```python
from build123d import *

# Parameters (mm, degrees)
SKETCH_1_R        = 80
SKETCH_1_R_2      = 43
EXTRUDE_1_DEPTH   = 70
SKETCH_1_R_3      = 50
SKETCH_1_R_4      = 22.5
EXTRUDE_1_2_DEPTH = 70
EXTRUDE_START     = -52.5
EXTRUDE_2_DEPTH   = 35


with BuildPart() as part:
    # Sketch 1 → Extrude 1 (new body)
    with BuildSketch(Plane(origin=(0, 0, 0), x_dir=(1, 0, 0), z_dir=(0, 1, 0))):
        with Locations(Location((-122.899042893, 0, 0), (0, 0, 270))):
            Circle(SKETCH_1_R)
        with Locations(Location((-122.899042893, 0, 0), (0, 0, 270))):
            Circle(SKETCH_1_R_2, mode=Mode.SUBTRACT)
    extrude(amount=EXTRUDE_1_DEPTH)



with BuildPart() as body_2:
    # Sketch 1 → Extrude 1 2 (new body)
    with BuildSketch(Plane(origin=(0, 0, 0), x_dir=(1, 0, 0), z_dir=(0, 1, 0))):
        with Locations(Location((107.100957107, 0, 0), (0, 0, 270))):
            Circle(SKETCH_1_R_3)
        with Locations(Location((107.100957107, 0, 0), (0, 0, 270))):
            Circle(SKETCH_1_R_4, mode=Mode.SUBTRACT)
    extrude(amount=EXTRUDE_1_2_DEPTH)


with BuildPart() as part_1:
    add(part.part)

    add(body_2.part)  # Extrude 2 merges body 2
    # Sketch 2 → Extrude 2 (add)
    with BuildSketch(Plane(origin=(0, 70, 0), x_dir=(1, 0, 0), z_dir=(0, 1, 0)).offset(EXTRUDE_START)):
        with BuildLine():
            Line((-112.464260284, 79.316551311), (113.622696237, 49.57284457))
            ThreePointArc((113.622696237, 49.57284457), (61.083229888, 19.554252264), (75.941536817, -39.10358714))
            ThreePointArc((75.941536817, -39.10358714), (4.230318414, -17.752822315), (-62.222714391, -52.138116186))
            ThreePointArc((-62.222714391, -52.138116186), (-48.171003091, 28.560813493), (-112.464260284, 79.316551311))
        make_face()
    extrude(amount=EXTRUDE_2_DEPTH)


solid = part_1.part
```
The listing builds one solid part. Answer for the finished solid, in the listing's coordinates (mm). A direction names the side the tool comes from. Coordinates: 2 decimals unless noted, no trailing zeros. Loops run counter-clockwise (first coordinate to the right, second up) from the corner with the lowest first, then second, coordinate; pieces in that order, holes last. Notation, with made-up numbers: (61, 16.25) -> (89, 16.25) arc R22 ccw to (89, 30.25) -> close; hole circle Ø6 at (5, 66.25). An arc over 180 degrees is marked (long way). Use one line per item in the form item = value. Start each with the question number.
Item 1: Consider L1, parallel to X at y = 47, z = 0; L2, parallel to X at y = 13, z = 5; L3, parallel to Z at x = 132.5, y = 61. Determine where each line is inside the solid, lowest interval first. Write a range as [from, to].
Item 2: The part is cut by section C-C on y = 60. Determine the outline of the cut face in (x, z), then the cut area to 3 significant figures.
Item 3: Flat-ended cylindrical pins translate along their axes: pin 1 Ø8 at (x, y) = (-107.5, 12.5) entering from +Z; pin 2 Ø1 at (y, z) = (16, -45.5) entering from -X; pin 3 Ø6 at (y, z) = (23.5, -52) entering from -X; pin 4 Ø5 at (x, z) = (104, -55) entering from -Y. Find the tip coordinate at first contact, or state that the pin passes through.
Item 4: The mould has two halves that part along X. Classify faces 1 (the face through (-1.003, 34.755, -64.653)), 2 (the face through (-157, 0, 34)), 3 (the face through (1, 17.5, -24)): released by +X, released by -X, zero draft, split by the parting line, or undercut.
Item 5: The part is cut by section D-D on z = -60.5. Determine the outline of the cut face in (x, y), then the cut area to 3 significant figures.
Item 6: The part is cut by section B-B on x = 124. Determine the outline of the cut face in (y, z), then the cut area to 3 significant figures.
Item 7: A tool of negligible diameter and unlimited length cuts with its end or side. For faces 4 (the face through (149.26, 34.51, 26.88)), 5 (the face through (5.3, 34.755, 17.658)), from which of +Z, -Z, +X, -X, +Y, -Y can it reach the whole face along a straight path? Write none if from no direction.
Item 8: The part is cut by section A-A on z = 0. Determine the outline of the cut face in (x, y).
Answer key:
q1.L1 = [-202.9, -165.9], [-79.9, 84.6], [129.6, 157.1]
q1.L2 = [-202.74, -165.61], [-80.19, -43.06], [57.35, 85.16], [129.04, 156.85]
q1.L3 = [-43.07, 43.07]
q2.outline = circle Ø160 at (-122.9, 0); circle Ø100 at (107.1, 0); hole circle Ø86 at (-122.9, 0); hole circle Ø45 at (107.1, 0)
q2.area = 20,600 mm2
q3.pin_1 = 79.18
q3.pin_2 = -189.04
q3.pin_3 = -186.14
q3.pin_4 = through
q4.face_1 = released by +X
q4.face_2 = zero draft
q4.face_3 = undercut
q5.outline = (-175.24, 0) -> (-70.56, 0) -> (-70.56, 17.5) -> (30.56, 17.5) -> (30.56, 52.5) -> (-70.56, 52.5) -> (-70.56, 70) -> (-175.24, 70) -> close
q5.area = 10,900 mm2
q6.outline = (0, -47.06) -> (70, -47.06) -> (70, -14.86) -> (0, -14.86) -> close; (0, 14.86) -> (70, 14.86) -> (70, 47.06) -> (0, 47.06) -> close
q6.area = 4,510 mm2
q7.face_4 = none
q7.face_5 = +Z, +Y, -Y
q8.outline = (-202.9, 0) -> (-165.9, 0) -> (-165.9, 70) -> (-202.9, 70) -> close; (-79.9, 0) -> (-42.9, 0) -> (-42.9, 17.5) -> (57.1, 17.5) -> (57.1, 0) -> (84.6, 0) -> (84.6, 70) -> (57.1, 70) -> (57.1, 52.5) -> (-42.9, 52.5) -> (-42.9, 70) -> (-79.9, 70) -> close; (129.6, 0) -> (157.1, 0) -> (157.1, 70) -> (129.6, 70) -> close
